The model under review builds one solid part; all positions refer to its coordinate system, in mm. A direction names the side the tool comes from. Round coordinates to 2 decimals unless told otherwise and drop trailing zeros. Loops run counter-clockwise (first coordinate to the right, second up) from the corner with the lowest first, then second, coordinate; pieces in that order, holes last. Notation, with made-up numbers: (22, 55.5) -> (60, 55.5) arc R16 ccw to (60, 70.5) -> close; hole circle Ø9 at (18.25, 83). An arc over 180 degrees is marked (long way). Return JSON: item names as keys, results as strings. Group by question number.
```python
from build123d import *

# Parameters (mm, degrees)
F0_R     = 9
F1_DEPTH = 16
F2_DEPTH = 4
F3_DEPTH = 15
F4_R     = 5
F5_R     = 1
F6_SIZE2 = 25
F6_SIZE  = 1.8


with BuildPart() as f1:
    # F0 (on Top) → F1 (new body)
    with BuildSketch(Plane.XY):
        Circle(F0_R)
        Polygon((-4.85, 4.85), (0, 4.85), (4.85, 4.85), (4.85, -4.85), (0, -4.85), (-4.85, -4.85), align=None, mode=Mode.SUBTRACT)
        with BuildLine():
            Line((3.4119543857, 2.130107217), (3.5507041555, 2.05))
            Line((3.5507041555, 2.05), (3.5507041555, -2.05))
            Line((3.5507041555, -2.05), (3.4119543857, -2.130107217))
            ThreePointArc((3.4119543857, -2.130107217), (2.1816994225, -4.0868207157), (0, -4.85))
            Line((0, -4.85), (4.85, -4.85))
            Line((4.85, -4.85), (4.85, 4.85))
            Line((4.85, 4.85), (0, 4.85))
            ThreePointArc((0, 4.85), (2.1816994225, 4.0868207157), (3.4119543857, 2.130107217))
        make_face()
        with BuildLine():
            ThreePointArc((-3.4119543857, 2.130107217), (-2.1816994225, 4.0868207157), (0, 4.85))
            Line((0, 4.85), (-4.85, 4.85))
            Line((-4.85, 4.85), (-4.85, -4.85))
            Line((-4.85, -4.85), (0, -4.85))
            ThreePointArc((0, -4.85), (-2.1816994225, -4.0868207157), (-3.4119543857, -2.130107217))
            Line((-3.4119543857, -2.130107217), (-3.5507041555, -2.05))
            Line((-3.5507041555, -2.05), (-3.5507041555, 2.05))
            Line((-3.5507041555, 2.05), (-3.4119543857, 2.130107217))
        make_face()
    extrude(amount=F1_DEPTH)

    # F0 (on Top) → F2 (join)
    with BuildSketch(Plane.XY):
        with BuildLine():
            ThreePointArc((0, -4.85), (2.1816994225, -4.0868207157), (3.4119543857, -2.130107217))
            Line((3.4119543857, -2.130107217), (0, -4.1))
            Line((0, -4.1), (-3.4119543857, -2.130107217))
            ThreePointArc((-3.4119543857, -2.130107217), (-2.1816994225, -4.0868207157), (0, -4.85))
        make_face()
        with BuildLine():
            Line((0, 4.1), (3.4119543857, 2.130107217))
            ThreePointArc((3.4119543857, 2.130107217), (2.1816994225, 4.0868207157), (0, 4.85))
            ThreePointArc((0, 4.85), (-2.1816994225, 4.0868207157), (-3.4119543857, 2.130107217))
            Line((-3.4119543857, 2.130107217), (0, 4.1))
        make_face()
    extrude(amount=F2_DEPTH)

    # F0 (on Top) → F3 (join)
    with BuildSketch(Plane.XY):
        Circle(F0_R)
        Polygon((-4.85, 4.85), (0, 4.85), (4.85, 4.85), (4.85, -4.85), (0, -4.85), (-4.85, -4.85), align=None, mode=Mode.SUBTRACT)
    extrude(amount=-F3_DEPTH)

    # F4
    f4_edges = [f1.edges().sort_by_distance(p)[0] for p in [
        (0, -4.1, 2),
        (0, 4.1, 2),
    ]]
    fillet(f4_edges, radius=F4_R)

    # F5
    f5_edges = [f1.edges().sort_by_distance(p)[0] for p in [
        (-4.85, -4.85, -7.5),
        (4.85, -4.85, -7.5),
        (4.85, 4.85, -7.5),
        (-4.85, 4.85, -7.5),
        (0, -4.85, 0),
        (-4.85, 0, 0),
        (0, 4.85, 0),
        (4.85, 0, 0),
    ]]
    fillet(f5_edges, radius=F5_R)

    # F6
    f6_edges = [f1.edges().sort_by_distance(p)[0] for p in [
        (-9, 0, 16),
    ]]
    f6_side = f1.faces().sort_by_distance((3.608608, 2.310508, 16))[0]
    chamfer(f6_edges, length=F6_SIZE, length2=F6_SIZE2, reference=f6_side)


solid = f1.part
```
1. For P1, Ø3, axis at x = 0.5, y = 3, coming from the +Z side; P2, Ø2.5, axis at x = -1, y = 0, coming from the -Z side; P3, Ø1.2, axis at y = -0.5, z = 8.5, coming from the +X side; P4, Ø1.5, axis at y = 2.5, z = 2, coming from the -X side, all flat-tipped, find the tip position at first contact; note any pin that passes through.
2. We need section B-B, the plane y = 0. Write out the cut boundary in (x, z), then the cut area to 3 significant figures.
3. Tool access review of faces 1 (the face through (-3.551, 0, 8)), 2 (the face through (0, -4.85, -8)), 3 (the face through (0, 4, 4)): name each direction out of +Z, -Z, +X, -X, +Y, -Y from which nothing blocks a thin tool from reaching the whole face with its end or side.
4. We need section C-C, the plane z = 10. Write out the cut boundary in (x, y).
5. We need section A-A, the plane z = -11.5. Write out the cut boundary in (x, y), then the cut area to 3 significant figures.
6. Wall thickness on line 1 (X direction, y = -1.25, z = -10.5); line 2 (X direction, y = 3.75, z = 4.5); line 3 (X direction, y = -5.25, z = 7): over which ranges is each line inside the solid? List them lowest first.
7. Draft analysis for pull direction Y (two halves, no side actions). For faces 4 (the face through (-1.172, 8.923, -11.958)), 5 (the face through (3.1, 3.3, 16)), 6 (the face through (-0.037, 3.326, 2.028)), state which applies: pulls with the +Y half, pulls with the -Y half, needs draft (parallel to the pull), parting line crosses it, or undercut.
Check sheet entries:
{
 "1": {"P1": "stops at z = 4", "P2": "passes through", "P3": "stops at x = 7.78", "P4": "stops at x = -8.03"},
 "2": {"outline": "(-9, -15) -> (-4.85, -15) -> (-4.85, -1) arc R1 cw to (-3.85, 0) -> (-3.55, 0) -> (-3.55, 16) -> (-7.2, 16) -> (-9, -9) -> close; (3.55, 0) -> (3.85, 0) arc R1 cw to (4.85, -1) -> (4.85, -15) -> (9, -15) -> (9, -9) -> (7.2, 16) -> (3.55, 16) -> close", "area": "254 mm²"},
 "3": {"face 1": "+Z, -Z", "face 2": "-Z", "face 3": "+Z"},
 "4": {"outline": "circle Ø15.26 at (0, 0); hole (-3.55, -2.05) -> (-3.41, -2.13) arc R3.5 ccw to (3.41, -2.13) -> (3.55, -2.05) -> (3.55, 2.05) -> (3.41, 2.13) arc R3.5 ccw to (-3.41, 2.13) -> (-3.55, 2.05) -> close"},
 "5": {"outline": "circle Ø18 at (0, 0); hole (-4.85, -3.85) arc R1 ccw to (-3.85, -4.85) -> (3.85, -4.85) arc R1 ccw to (4.85, -3.85) -> (4.85, 3.85) arc R1 ccw to (3.85, 4.85) -> (-3.85, 4.85) arc R1 ccw to (-4.85, 3.85) -> close", "area": "161 mm²"},
 "6": {"line 1": "x = -8.91 to -4.85, 4.85 to 8.91", "line 2": "x = -7.1 to -2.55, 2.55 to 7.1", "line 3": "x = -5.83 to 5.83"},
 "7": {"face 4": "parting line crosses it", "face 5": "needs draft", "face 6": "undercut"}
}
